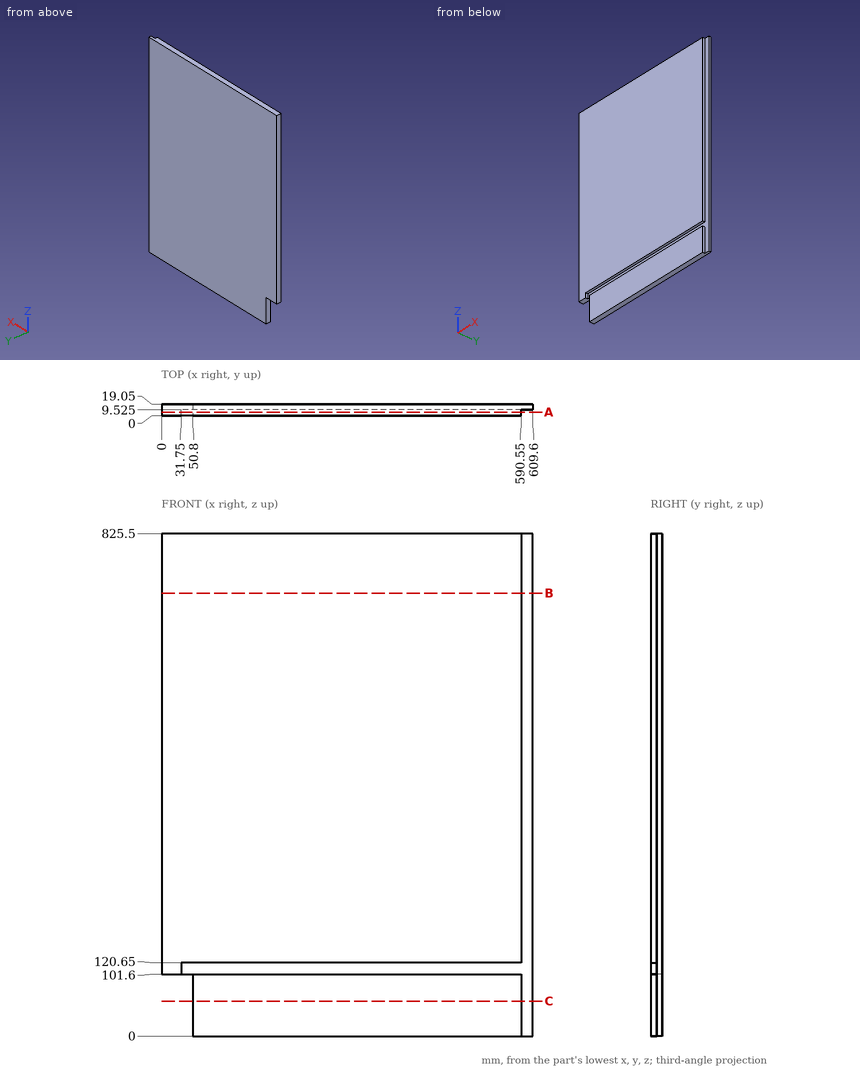
The figure shows three views and two pictorial views of one solid part (mm, origin at its lowest corner). Answer the questions. Give positions to 0.01 mm unless a question says otherwise; leave off trailing zeros. Write each loop counter-clockwise with the first axis right and the second up, starting at its lowest first coordinate (ties: lowest second). Pieces come first, ordered by that corner, then holes.
Q1. The part is cut by section C-C on z = 57.5. Give the vertices of the cut face in (x, y) (3 decimals), and give its area (3 significant figures).
Answer:
outline: (50.8, 0) - (590.55, 0) - (590.55, 9.525) - (609.6, 9.525) - (609.6, 19.05) - (50.8, 19.05) - close
area: 10,500 mm2
Q2. Straight lines are drawn through the part: L1, parallel to Z at x = 344, y = 2.5; L2, parallel to X at y = 4, z = 114; L3, parallel to Y at x = 127, z = 105 (3 decimals). For each, find the intervals that lie inside material, in ascending order.
Answer:
L1: z = 0 to 101.6, 120.65 to 825.5
L2: x = 0 to 31.75
L3: y = 9.525 to 19.05
Q3. The part is cut by section B-B on z = 727.5. Give the vertices of the cut face in (x, y) (3 decimals), and give its area (3 significant figures).
Answer:
outline: (0, 0) - (590.55, 0) - (590.55, 9.525) - (609.6, 9.525) - (609.6, 19.05) - (0, 19.05) - close
area: 11,400 mm2
Q4. The part is cut by section A-A on y = 5.5. Give the vertices of the cut face in (x, z), and give its area (3 significant figures).
Answer:
outline: (0, 101.6) - (31.75, 101.6) - (31.75, 120.65) - (590.55, 120.65) - (590.55, 825.5) - (0, 825.5) - close; (50.8, 0) - (590.55, 0) - (590.55, 101.6) - (50.8, 101.6) - close
area: 472,000 mm2
Q5. Given pin 1 (7.5 mm diameter, centred on y = 4, z = 455.5, fed in from +X); pin 2 (3 mm diameter, centred on y = 6, z = 109, fed in from +X); pin 3 (5.5 mm diameter, centred on x = 30, y = 12.5, fed in from -Z), each flat-ended and moving along its own axis, determine where each tip first touches the part or whether it passes through.
Answer:
pin 1: stops at x = 590.55
pin 2: stops at x = 31.75
pin 3: stops at z = 101.6
